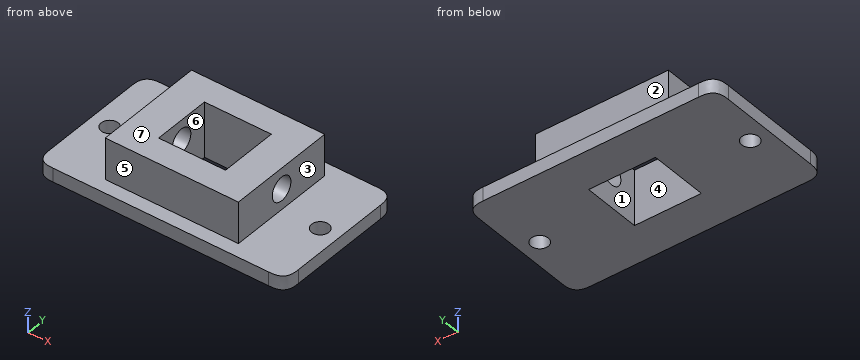
from build123d import *

# Parameters (mm, degrees)
SKETCH1_W           = 45
SKETCH1_H           = 25
SKETCH1_W_2         = 12.1
SKETCH1_H_2         = 10.6
BOSS_EXTRUDE1_DEPTH = 2.5
SKETCH2_W           = 12.1
SKETCH2_H           = 7.2
BOSS_EXTRUDE2_DEPTH = 7.5
BOSS_EXTRUDE3_START = 6.05
SKETCH3_W           = 7.5
SKETCH3_H           = 25
SKETCH3_R           = 2.15
BOSS_EXTRUDE3_DEPTH = 6
BOSS_EXTRUDE4_START = -14.05
SKETCH3_2_W         = 7.5
SKETCH3_2_H         = 25
SKETCH3_2_R         = 2.15
BOSS_EXTRUDE4_DEPTH = 8
SKETCH5_R           = 1.55
CUT_EXTRUDE1_DEPTH  = 10
FILLET1_SIZE        = 3
SKETCH6_OUTSIDE_W   = 57.488
SKETCH6_OUTSIDE_H   = 37.488
SKETCH6_OUTSIDE_W_2 = 24.1
SKETCH6_OUTSIDE_H_2 = 19.953815678
CUT_EXTRUDE2_DEPTH  = 7.5


with BuildPart() as part:
    # Sketch1 → Boss-Extrude1 (new body)
    with BuildSketch(Plane.XY):
        Rectangle(SKETCH1_W, SKETCH1_H)
        Rectangle(SKETCH1_W_2, SKETCH1_H_2, mode=Mode.SUBTRACT)
    extrude(amount=BOSS_EXTRUDE1_DEPTH)

    # Sketch2 → Boss-Extrude2 (add)
    with BuildSketch(Plane.XY.offset(2.5)):
        with Locations((0, -8.9)):
            Rectangle(SKETCH2_W, SKETCH2_H)
        with Locations((0, 8.9)):
            Rectangle(SKETCH2_W, SKETCH2_H)
    extrude(amount=BOSS_EXTRUDE2_DEPTH)

    # Sketch3 → Boss-Extrude3 (add)
    with BuildSketch(Plane(origin=(0, 0, 0), x_dir=(0, 0, -1), z_dir=(1, 0, 0)).offset(BOSS_EXTRUDE3_START)):
        with Locations((-6.25, 0)):
            Rectangle(SKETCH3_W, SKETCH3_H)
        with Locations(Location((-6.25, 0, 0), (0, 0, 180))):
            Circle(SKETCH3_R, mode=Mode.SUBTRACT)
    extrude(amount=BOSS_EXTRUDE3_DEPTH)

    # Sketch3<2> → Boss-Extrude4 (add)
    with BuildSketch(Plane(origin=(0, 0, 0), x_dir=(0, 0, -1), z_dir=(1, 0, 0)).offset(BOSS_EXTRUDE4_START)):
        with Locations((-6.25, 0)):
            Rectangle(SKETCH3_2_W, SKETCH3_2_H)
        with Locations(Location((-6.25, 0, 0), (0, 0, 180))):
            Circle(SKETCH3_2_R, mode=Mode.SUBTRACT)
    extrude(amount=BOSS_EXTRUDE4_DEPTH)

    # Sketch5 → Cut-Extrude1 (cut)
    with BuildSketch(Plane(origin=(0, 0, 0), x_dir=(-1, 0, 0), z_dir=(0, 0, -1))):
        with Locations((-19.05, 0)):
            Circle(SKETCH5_R)
        with Locations(Location((19.05, 0, 0), (0, 0, 180))):
            Circle(SKETCH5_R)
    extrude(amount=-CUT_EXTRUDE1_DEPTH, mode=Mode.SUBTRACT)

    # Fillet1
    # a fillet whose section is not a circle: 3 mm, written as the material it takes off along each edge
    with BuildSketch(Plane(origin=(-22.5, -12.5, -7.5), x_dir=(0, 1, 0), z_dir=(0, 0, 1)), Plane(origin=(-22.5, 12.5, -7.5), x_dir=(1, 0, 0), z_dir=(0, 0, 1))) as fillet1_piece_1:
        with BuildLine():
            add(Edge.make_bspline([(FILLET1_SIZE, 0), (FILLET1_SIZE * 0.831801948466, 0), (FILLET1_SIZE * 0.663603896932, 0), (FILLET1_SIZE * 0.292893218813, -FILLET1_SIZE * 0.0716919198361), (FILLET1_SIZE * 0.0716919198361, -FILLET1_SIZE * 0.292893218813), (0, -FILLET1_SIZE * 0.663603896932), (0, -FILLET1_SIZE * 0.831801948466), (0, -FILLET1_SIZE)], knots=[0, 0, 0, 0, 0, 0, 0.5, 0.5, 1, 1, 1, 1, 1, 1], degree=5))
            Line((0, -FILLET1_SIZE), (0, 0))
            Line((0, 0), (FILLET1_SIZE, 0))
        make_face()
    extrude(amount=17.5, mode=Mode.SUBTRACT)
    with BuildSketch(Plane(origin=(22.5, -12.5, -7.5), x_dir=(0, 1, 0), z_dir=(0, 0, 1)), Plane(origin=(22.5, 12.5, -7.5), x_dir=(-1, 0, 0), z_dir=(0, 0, 1))) as fillet1_piece_2:
        with BuildLine():
            add(Edge.make_bspline([(FILLET1_SIZE, 0), (FILLET1_SIZE * 0.831801948466, 0), (FILLET1_SIZE * 0.663603896932, 0), (FILLET1_SIZE * 0.292893218813, FILLET1_SIZE * 0.0716919198361), (FILLET1_SIZE * 0.0716919198361, FILLET1_SIZE * 0.292893218813), (0, FILLET1_SIZE * 0.663603896932), (0, FILLET1_SIZE * 0.831801948466), (0, FILLET1_SIZE)], knots=[0, 0, 0, 0, 0, 0, 0.5, 0.5, 1, 1, 1, 1, 1, 1], degree=5))
            Line((0, FILLET1_SIZE), (0, 0))
            Line((0, 0), (FILLET1_SIZE, 0))
        make_face()
    extrude(amount=17.5, mode=Mode.SUBTRACT)

    # Sketch6 outside → Cut-Extrude2 (cut)
    with BuildSketch(Plane.XY.offset(10)):
        Rectangle(SKETCH6_OUTSIDE_W, SKETCH6_OUTSIDE_H)
        Rectangle(SKETCH6_OUTSIDE_W_2, SKETCH6_OUTSIDE_H_2, mode=Mode.SUBTRACT)
    extrude(amount=-CUT_EXTRUDE2_DEPTH, mode=Mode.SUBTRACT)


solid = part.part
Input: part model. Units: mm. Frame: model coordinates. Face numbers are marked on the shaded views. A direction names the side the tool comes from. Coordinates: 2 decimals unless noted, no trailing zeros. Order: outer loops, then holes, each group sorted by start corner. A loop starts at its lowest first (then second) coordinate and runs counter-clockwise, first axis right, second up. Notation, with made-up numbers: M 50.25,34 L 99.25,34 A23 cw 99.25,42 Z; hole C -3,28.5 d10. An arc over 180 degrees is marked long. Answer as CSV lines item,"result".
1. Access query for the marked faces 5, 6 and 7. Directions: +Z, -Z, +X, -X, +Y, -Y. A direction counts if a zero-diameter tool reaches every point of the face in a straight line with its end or side. Return the directions, or none.
Reported:
face 5,"+Z, +X, -X, -Y"
face 6,"+Z, -Z"
face 7,"+Z, +X, -X, +Y, -Y"
2. First-contact query: P1, Ø4, axis at y = 0, z = 6.25, coming from the -X side; P2, Ø4, axis at y = -4.5, z = 7, coming from the -X side; P3, Ø4, axis at x = -4, z = 6, coming from the -Y side; P4, Ø1, axis at x = -3, z = 5.5, coming from the +Y side. Flat tips, straight axial feed; report the tip coordinate or a pass-through.
Reported:
P1,"through"
P2,"x = -12.05"
P3,"y = -9.98"
P4,"y = 9.98"
3. Section D-D (z = 9). Return the cut outline in (x, y), then the cut area to 3 significant figures.
Reported:
outline,"M -12.05,-9.98 L 12.05,-9.98 L 12.05,9.98 L -12.05,9.98 Z; hole M -6.05,-5.3 L 6.05,-5.3 L 6.05,5.3 L -6.05,5.3 Z"
area,"353 mm2"
4. Section B-B (x = -19.05). Return the cut outline in (y, z).
Reported:
outline,"M -12.5,0 L -1.55,0 L -1.55,2.5 L -12.5,2.5 Z; M 1.55,0 L 12.5,0 L 12.5,2.5 L 1.55,2.5 Z"
5. Section C-C (z = 6.25). Return the cut outline in (x, y).
Reported:
outline,"M -12.05,-9.98 L 12.05,-9.98 L 12.05,-2.15 L 6.05,-2.15 L 6.05,-5.3 L -6.05,-5.3 L -6.05,-2.15 L -12.05,-2.15 Z; M -12.05,2.15 L -6.05,2.15 L -6.05,5.3 L 6.05,5.3 L 6.05,2.15 L 12.05,2.15 L 12.05,9.98 L -12.05,9.98 Z"
6. Section A-A (y = 0). Return the cut outline in (x, z).
Reported:
outline,"M -22.5,0 L -20.6,0 L -20.6,2.5 L -22.5,2.5 Z; M -17.5,0 L -6.05,0 L -6.05,4.1 L -12.05,4.1 L -12.05,2.5 L -17.5,2.5 Z; M -12.05,8.4 L -6.05,8.4 L -6.05,10 L -12.05,10 Z; M 6.05,0 L 17.5,0 L 17.5,2.5 L 12.05,2.5 L 12.05,4.1 L 6.05,4.1 Z; M 6.05,8.4 L 12.05,8.4 L 12.05,10 L 6.05,10 Z; M 20.6,0 L 22.5,0 L 22.5,2.5 L 20.6,2.5 Z"
7. Material intervals for line 1 (Y direction, x = 8.5, z = 6.25); line 2 (X direction, y = 3.75, z = 8); line 3 (Y direction, x = -4, z = 2.25), sorted ascending. Write a range as from..to.
Reported:
line 1,"-9.98..-2.15, 2.15..9.98"
line 2,"-12.05..-6.05, 6.05..12.05"
line 3,"-12.5..-5.3, 5.3..12.5"
8. Pull-direction query (X, two-part tool) for the marked faces 1, 2, 3 and 4; classes: released by +X, released by -X, zero draft, split by the parting line, or undercut.
Reported:
face 1,"undercut"
face 2,"zero draft"
face 3,"released by +X"
face 4,"undercut"
